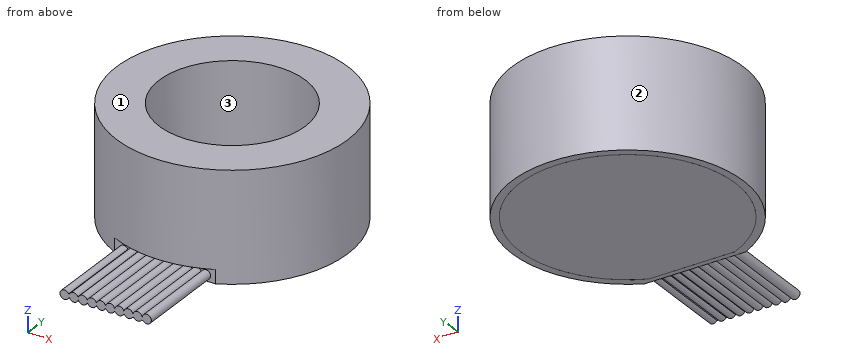
```python
from build123d import *

# Parameters (mm, degrees)
SKETCH_1_R          = 12.65
EXTRUDE_1_DEPTH     = 12
CUT_EXTRUDE_START   = 9
CUT_EXTRUDE_1_DEPTH = 9
CUT_EXTRUDE_2_DEPTH = 0.5
EXTRUDE_5_DEPTH     = 10
SKETCH_4_R          = 8
CUT_EXTRUDE_3_DEPTH = 10
CUT_EXTRUDE_4_DEPTH = 1


with BuildPart() as part:
    # 草图1 → 凸台-拉伸1 (new body)
    with BuildSketch(Plane.XY):
        Circle(SKETCH_1_R)
    extrude(amount=EXTRUDE_1_DEPTH)

    # 草图2 → 切除-拉伸1 (cut)
    with BuildSketch(Plane(origin=(0, 0, 1), x_dir=(-1, 0, 0), z_dir=(0, 0, -1)).offset(CUT_EXTRUDE_START)):
        with BuildLine():
            Line((0, -11.379520841), (-5.525305913, -11.379520841))
            ThreePointArc((-5.525305913, -11.379520841), (0, -12.65), (5.525305913, -11.379520841))
            Line((5.525305913, -11.379520841), (0, -11.379520841))
        make_face()
    extrude(amount=-CUT_EXTRUDE_1_DEPTH, mode=Mode.SUBTRACT)

    # 草图2<2> → 切除-拉伸2 (cut)
    with BuildSketch(Plane(origin=(0, 0, 1), x_dir=(-1, 0, 0), z_dir=(0, 0, -1))):
        with BuildLine():
            Line((0, -11.379520841), (-5.525305913, -11.379520841))
            ThreePointArc((-5.525305913, -11.379520841), (0, -12.65), (5.525305913, -11.379520841))
            Line((5.525305913, -11.379520841), (0, -11.379520841))
        make_face()
    extrude(amount=-CUT_EXTRUDE_2_DEPTH, mode=Mode.SUBTRACT)

    # 草图3 → 凸台-拉伸5 (add)
    with BuildSketch(Plane.XZ.offset(11.379520841)):
        with BuildLine():
            Line((-4.052610832, 0.723255308), (-3.95666659, 0.723255308))
            ThreePointArc((-3.95666659, 0.723255308), (-3.5, 1.019648763), (-3.04333341, 0.723255308))
            Line((-3.04333341, 0.723255308), (-2.964929601, 0.723255308))
            ThreePointArc((-2.964929601, 0.723255308), (-2.5, 1.039297525), (-2.035070399, 0.723255308))
            Line((-2.035070399, 0.723255308), (-1.972231454, 0.723255308))
            ThreePointArc((-1.972231454, 0.723255308), (-1.5, 1.058946288), (-1.027768546, 0.723255308))
            Line((-1.027768546, 0.723255308), (-0.97861614, 0.723255308))
            ThreePointArc((-0.97861614, 0.723255308), (-0.5, 1.07859505), (-0.02138386, 0.723255308))
            Line((-0.02138386, 0.723255308), (0.01588005, 0.723255308))
            ThreePointArc((0.01588005, 0.723255308), (0.5, 1.098243813), (0.98411995, 0.723255308))
            Line((0.98411995, 0.723255308), (1.011227359, 0.723255308))
            ThreePointArc((1.011227359, 0.723255308), (1.5, 1.117892575), (1.988772641, 0.723255308))
            Line((1.988772641, 0.723255308), (2.007401669, 0.723255308))
            ThreePointArc((2.007401669, 0.723255308), (2.5, 1.137541338), (2.992598331, 0.723255308))
            Line((2.992598331, 0.723255308), (3.00438383, 0.723255308))
            ThreePointArc((3.00438383, 0.723255308), (3.5, 1.1571901), (3.99561617, 0.723255308))
            Line((3.99561617, 0.723255308), (4.002159148, 0.723255308))
            ThreePointArc((4.002159148, 0.723255308), (4.983765438, 0.803215289), (4.088469212, 0.392862789))
            Line((4.088469212, 0.392862789), (3.924418511, 0.392862789))
            ThreePointArc((3.924418511, 0.392862789), (3.5, 0.1571901), (3.075581489, 0.392862789))
            Line((3.075581489, 0.392862789), (2.93604175, 0.392862789))
            ThreePointArc((2.93604175, 0.392862789), (2.5, 0.137541338), (2.06395825, 0.392862789))
            Line((2.06395825, 0.392862789), (1.946499267, 0.392862789))
            ThreePointArc((1.946499267, 0.392862789), (1.5, 0.117892575), (1.053500733, 0.392862789))
            Line((1.053500733, 0.392862789), (0.955871292, 0.392862789))
            ThreePointArc((0.955871292, 0.392862789), (0.5, 0.098243813), (0.044128708, 0.392862789))
            Line((0.044128708, 0.392862789), (-0.035776425, 0.392862789))
            ThreePointArc((-0.035776425, 0.392862789), (-0.5, 0.07859505), (-0.964223575, 0.392862789))
            Line((-0.964223575, 0.392862789), (-1.028389704, 0.392862789))
            ThreePointArc((-1.028389704, 0.392862789), (-1.5, 0.058946288), (-1.971610296, 0.392862789))
            Line((-1.971610296, 0.392862789), (-2.021923784, 0.392862789))
            ThreePointArc((-2.021923784, 0.392862789), (-2.5, 0.039297525), (-2.978076216, 0.392862789))
            Line((-2.978076216, 0.392862789), (-3.016341735, 0.392862789))
            ThreePointArc((-3.016341735, 0.392862789), (-3.5, 0.019648763), (-3.983658265, 0.392862789))
            Line((-3.983658265, 0.392862789), (-4.01161325, 0.392862789))
            ThreePointArc((-4.01161325, 0.392862789), (-4.996194464, 0.438428468), (-4.052610832, 0.723255308))
        make_face()
    extrude(amount=EXTRUDE_5_DEPTH)

    # 草图4 → 切除-拉伸3 (cut)
    with BuildSketch(Plane.XY.offset(12)):
        Circle(SKETCH_4_R)
    extrude(amount=-CUT_EXTRUDE_3_DEPTH, mode=Mode.SUBTRACT)

    # 草图5 → 切除-拉伸4 (cut)
    with BuildSketch(Plane(origin=(0, 0, 0), x_dir=(-1, 0, 0), z_dir=(0, 0, -1))):
        with BuildLine():
            Line((-4.710329459, -10.815249292), (4.710329459, -10.815249292))
            ThreePointArc((4.710329459, -10.815249292), (0, 11.796474934), (-4.710329459, -10.815249292))
        make_face()
        with BuildLine():
            Line((-4.711523736, -10.812427627), (4.711523736, -10.812427627))
            ThreePointArc((4.711523736, -10.812427627), (0, 11.794365057), (-4.711523736, -10.812427627))
        make_face(mode=Mode.SUBTRACT)
    extrude(amount=-CUT_EXTRUDE_4_DEPTH, mode=Mode.SUBTRACT)


solid = part.part
```
Check sheet for the modelled part. Datum: model origin and axes. Units: mm. Face numbers are marked on the shaded views. Coordinates: 2 decimals unless noted, no trailing zeros. Write each loop counter-clockwise with the first axis right and the second up, starting at its lowest first coordinate (ties: lowest second). Pieces come first, ordered by that corner, then holes. Notation, with made-up numbers: (-37.5, 63) -> (-12.5, 63) arc R30 ccw to (-12.5, 92) -> close; hole circle Ø9 at (-17.5, 73.5). An arc over 180 degrees is marked (long way). Use a Markdown table: item, result.
1. Scan lines: line 1 along Y through (x, z) = (0, 8.5); line 2 along X through (y, z) = (-0.5, 3.25); line 3 along Z through (x, y) = (0.25, 7.5). Record each from-to range of solid material in increasing order.
Reported:
| item | result |
|---|---|
| line 1 | y = -12.65 to -8, 8 to 12.65 |
| line 2 | x = -12.64 to -7.98, 7.98 to 12.64 |
| line 3 | z = 0 to 2 |
2. Release check for a two-part mould opening along Y. For the marked faces 1, 2 and 3 record: pulls with the +Y half, pulls with the -Y half, needs draft (parallel to the pull), parting line crosses it, or undercut.
Reported:
| item | result |
|---|---|
| face 1 | needs draft |
| face 2 | parting line crosses it |
| face 3 | undercut |
3. Sectioned sample at B-B (z = 9.75). Enter the section's corners in (x, y).
Reported:
| item | result |
|---|---|
| outline | circle Ø25.3 at (0, 0); hole circle Ø16 at (0, 0) |
4. Go/stop test with flat-tipped pins: pin 1 Ø0.6 at (x, y) = (2, -12) entering from -Z; pin 2 Ø2 at (x, z) = (-7.5, 10.5) entering from +Y; pin 3 Ø6 at (y, z) = (-8, 2) entering from +X. Record where each tip stops, or that it passes through.
Reported:
| item | result |
|---|---|
| pin 1 | stops at z = 0.16 |
| pin 2 | stops at y = 10.85 |
| pin 3 | stops at x = 11.62 |
